Source: CAD feature listing. Evaluate the final solid. Frame: model axes, mm. Round coordinates to 2 decimals unless told otherwise and drop trailing zeros. Loops run counter-clockwise (first coordinate to the right, second up) from the corner with the lowest first, then second, coordinate; pieces in that order, holes last. Notation, with made-up numbers: (64, -2) - (103, -2) arc R28 ccw to (103, 26) - close; hole circle Ø11 at (-39.75, 27.25). An arc over 180 degrees is marked (long way). One line per question, with ' | ' between items. Start each with the question number.
1. Ray query, line 1 (Z direction, x = 71.5, y = 0.9); line 2 (X direction, y = 0.8, z = -35.5); line 3 (Z direction, x = 47.5, y = 1.4). Return the intervals inside material, ascending.
2. Cut plane B-B (y = 0.85). State how many separate pieces and enclosed holes the cut face has, then the cut area to 3 significant figures.
3. Pin query (flat end, axial travel): pin 1 (7 mm diameter, centred on x = 51.9, z = -21.88, fed in from -Y); pin 2 (0.9 mm diameter, centred on x = 91.5, y = 1, fed in from -Z). Return the tip coordinate at first contact, or that it passes through.
4. Mould query, pull axis Z, two halves, no side actions, for faces 1 (the cylindrical face through (72.703, 0.913, -46.916)), 2 (the flat face through (49, 1.8, -50)), 3 (the cylindrical face through (42.105, 0.913, -75.727)). Classes: pulls with the +Z half, pulls with the -Z half, needs draft (parallel to the pull), parting line crosses it, or undercut.
5. Cut plane A-A (x = 70.5). Return loops of the section in (y, z), then the cut area to 3 significant figures.
6. Cut plane C-C (x = 37). Return loops of the section in (y, z).
7. Cut plane D-D (z = -91.5). Return loops of the section in (x, y), then the cut area to 3 significant figures.
```python
from build123d import *

# Parameters (mm, degrees)
SKETCH_1_W          = 99
SKETCH_1_H          = 99
EXTRUDE_1_DEPTH     = 1.8
SKETCH_2_R          = 3
SKETCH_2_R_2        = 3.197874374
CUT_EXTRUDE_1_DEPTH = 2.8
SKETCH_3_W          = 15
SKETCH_3_H          = 20
CUT_EXTRUDE_2_DEPTH = 2.8


with BuildPart() as part:
    # 草图1 → 凸台-拉伸1 (new body)
    with BuildSketch(Plane(origin=(0, 0, 0), x_dir=(1, 0, 0), z_dir=(0, 1, 0))):
        with Locations((49.5, 49.5)):
            Rectangle(SKETCH_1_W, SKETCH_1_H)
    extrude(amount=EXTRUDE_1_DEPTH)

    # 草图2 → 切除-拉伸1 (cut, through all)
    with BuildSketch(Plane(origin=(0, 1.8, 0), x_dir=(1, 0, 0), z_dir=(0, 1, 0))):
        with Locations((29.29818934, 71.224140528)):
            Circle(SKETCH_2_R)
        with Locations((45.102003727, 75.595349176)):
            Circle(SKETCH_2_R)
        with Locations((30.092218758, 60.228792633)):
            Circle(SKETCH_2_R)
        with Locations((35.605107574, 46.450435365)):
            Circle(SKETCH_2_R)
        with Locations((43.275213753, 34.342184277)):
            Circle(SKETCH_2_R)
        with Locations((56.937590385, 33.623111823)):
            Circle(SKETCH_2_R)
        with Locations((49.267484206, 46.806106819)):
            Circle(SKETCH_2_R)
        with Locations((64.847387383, 43.450435365)):
            Circle(SKETCH_2_R)
        with Locations((69.641203745, 56.633430361)):
            Circle(SKETCH_2_R)
        with Locations((57.65666284, 63.344773268)):
            Circle(SKETCH_2_R)
        with Locations((43.035522935, 57.112811997)):
            Circle(SKETCH_2_R)
        with Locations((43.275213753, 65.981372267)):
            Circle(SKETCH_2_R)
        with Locations((59.813880203, 73.172096811)):
            Circle(SKETCH_2_R)
        with Locations((69.401512927, 31.945276096)):
            Circle(SKETCH_2_R)
        with Locations((31.05098203, 29.068986279)):
            Circle(SKETCH_2_R)
        with Locations((51.904083205, 21.878261736)):
            Circle(SKETCH_2_R)
        with Locations((21.942730942, 39.13600064)):
            Circle(SKETCH_2_R)
        with Locations((21.942730942, 51.483942546)):
            Circle(SKETCH_2_R)
        with Locations((74.914401743, 44.888580274)):
            Circle(SKETCH_2_R)
        with Locations((64.98656548, 22.175939833)):
            Circle(SKETCH_2_R)
        with Locations((37.043252483, 22.07613611)):
            Circle(SKETCH_2_R_2)
        with Locations((72.038111926, 68.13858963)):
            Circle(SKETCH_2_R)
        with Locations((57.177281203, 52.079304817)):
            Circle(SKETCH_2_R)
    extrude(amount=-CUT_EXTRUDE_1_DEPTH, mode=Mode.SUBTRACT)

    # 草图3 → 切除-拉伸2 (cut, through all)
    with BuildSketch(Plane(origin=(0, 1.8, 0), x_dir=(1, 0, 0), z_dir=(0, 1, 0))):
        with Locations((91.5, 89)):
            Rectangle(SKETCH_3_W, SKETCH_3_H)
    extrude(amount=-CUT_EXTRUDE_2_DEPTH, mode=Mode.SUBTRACT)


solid = part.part
```
Answers follow:
1) line 1: z = -99 to -71.09, -65.19 to -58.99, -54.28 to -34.09, -29.8 to 0 | line 2: x = 0 to 40.51, 46.04 to 54.6, 59.28 to 99 | line 3: z = -99 to -77.4, -73.79 to -49.23, -44.38 to 0
2) separate pieces: 1 | enclosed holes: 23 | area: 8,850 mm2
3) pin 1: stops at y = 0 | pin 2: stops at z = -79
4) face 1: undercut | face 2: needs draft | face 3: undercut
5) outline: (0, -99) - (1.8, -99) - (1.8, -70.71) - (0, -70.71) - close; (0, -65.56) - (1.8, -65.56) - (1.8, -59.51) - (0, -59.51) - close; (0, -53.76) - (1.8, -53.76) - (1.8, -34.74) - (0, -34.74) - close; (0, -29.15) - (1.8, -29.15) - (1.8, 0) - (0, 0) - close | area: 149 mm2
6) outline: (0, -99) - (1.8, -99) - (1.8, -49.11) - (0, -49.11) - close; (0, -43.79) - (1.8, -43.79) - (1.8, -25.27) - (0, -25.27) - close; (0, -18.88) - (1.8, -18.88) - (1.8, 0) - (0, 0) - close
7) outline: (0, 0) - (84, 0) - (84, 1.8) - (0, 1.8) - close | area: 151 mm2
